Here's how the part is built. I have some questions about the finished solid (model axes, mm). Face numbers are marked on the shaded views. Round coordinates to 2 decimals unless told otherwise and drop trailing zeros. Write each loop counter-clockwise with the first axis right and the second up, starting at its lowest first coordinate (ties: lowest second). Pieces come first, ordered by that corner, then holes. Notation, with made-up numbers: (30, 81) -> (57, 81) arc R19 ccw to (57, 88) -> close; hole circle Ø7 at (21, 71.25). An arc over 180 degrees is marked (long way). Answer in a Markdown table with one row per item.
from build123d import *

# Parameters (mm, degrees)
CYLINDER_R       = 1.2
CYLINDER_DEPTH   = 10
ARRAY001_X_COUNT = 2
ARRAY001_X_PITCH = 29.6
ARRAY001_Y_COUNT = 2
ARRAY001_Y_PITCH = 17.8
BOX003_W         = 23.6
BOX003_H         = 11.8
BOX003_DEPTH     = 10
BOX002_W         = 35.6
BOX002_H         = 23.8
BOX002_DEPTH     = 2.5
BOX017_W         = 2.5
BOX017_H         = 23.8
BOX017_DEPTH     = 1.5
BOX005_W         = 35.6
BOX005_H         = 2.5
BOX005_DEPTH     = 1.5


with BuildPart() as bolt_hole_array_clone:
    # Cylinder → Cylinder (new body)
    with BuildSketch(Plane.XY):
        Circle(CYLINDER_R)
    extrude(amount=CYLINDER_DEPTH)

    # Array001 X: bolt hole array clone ×2


with BuildPart() as bolt_hole_array_clone_1:
    add(bolt_hole_array_clone.part)
    with Locations(*[(i * ARRAY001_X_PITCH, 0, 0) for i in range(1, ARRAY001_X_COUNT)]):
        add(bolt_hole_array_clone.part)

    # Array001 Y: bolt hole array clone ×2


with BuildPart() as bolt_hole_array_clone_2:
    add(bolt_hole_array_clone_1.part)
    with Locations(*[(0, i * ARRAY001_Y_PITCH, 0) for i in range(1, ARRAY001_Y_COUNT)]):
        add(bolt_hole_array_clone_1.part)


with BuildPart() as bolt_hole_array_clone_3:
    # Array001 placement: moved
    add(bolt_hole_array_clone_2.part.moved(Location((3, 3, 0))))


with BuildPart() as mesh_extraction_fusion:
    # Box003 → Box003 (new body)
    with BuildSketch(Plane(origin=(6, 6, 0), x_dir=(1, 0, 0), z_dir=(0, 0, 1))):
        with Locations((11.8, 5.9)):
            Rectangle(BOX003_W, BOX003_H)
    extrude(amount=BOX003_DEPTH)

    # Fusion003: union bolt hole array clone
    add(bolt_hole_array_clone_3.part)


with BuildPart() as mesh_border_cut:
    # Box002 → Box002 (new body)
    with BuildSketch(Plane.XY):
        with Locations((17.8, 11.9)):
            Rectangle(BOX002_W, BOX002_H)
    extrude(amount=BOX002_DEPTH)

    # Cut001: cut mesh extraction fusion
    add(mesh_extraction_fusion.part, mode=Mode.SUBTRACT)


with BuildPart() as obj1:
    # Box017 → Box017 (new body)
    with BuildSketch(Plane.XY):
        with Locations((1.25, 11.9)):
            Rectangle(BOX017_W, BOX017_H)
    extrude(amount=BOX017_DEPTH)


with BuildPart() as obj1_1:
    # Array011 placement: moved
    add(obj1.part.moved(Location((16.55, 0, 0))))


with BuildPart() as x_mesh_holder_fusion:
    # Box005 → Box005 (new body)
    with BuildSketch(Plane.XY):
        with Locations((17.8, 1.25)):
            Rectangle(BOX005_W, BOX005_H)
    extrude(amount=BOX005_DEPTH)


with BuildPart() as x_mesh_holder_fusion_1:
    # Array002 placement: moved
    add(x_mesh_holder_fusion.part.moved(Location((0, 10.65, 0))))

    # Fusion001: union mesh border cut, obj1
    add(mesh_border_cut.part)
    add(obj1_1.part)


solid = x_mesh_holder_fusion_1.part
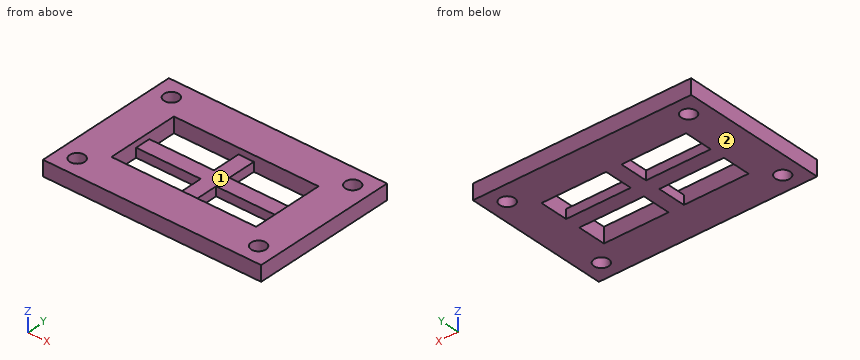
1) I want a section at C-C, the plane z = 0.45. Count the separate pieces of the cut face and the enclosed holes in it, and give its area (3 significant figures).
Response:
| item | result |
|---|---|
| separate pieces | 1 |
| enclosed holes | 8 |
| area | 633 mm^2 |
2) We'd pull the mould along Y, two halves only. Please class the marked faces 1 and 2: +Y half, -Y half, draft (parallel to the pull), parting line (faces both ways), or undercut.
Response:
| item | result |
|---|---|
| face 1 | undercut |
| face 2 | draft |
3) I need wall thicknesses on line 1 (Y direction, x = 12, z = 0.9); line 2 (X direction, y = 3, z = 1); line 3 (X direction, y = 6.5, z = 0.4). Which ranges of each line are inside material? Lowest first, please. Write a range as [from, to].
Response:
| item | result |
|---|---|
| line 1 | y = [0, 6], [10.65, 13.15], [17.8, 23.8] |
| line 2 | x = [0, 1.8], [4.2, 31.4], [33.8, 35.6] |
| line 3 | x = [0, 6], [16.55, 19.05], [29.6, 35.6] |
4) For pin 1 (3 mm diameter, centred on x = 32.6, y = 20.8, fed in from -Z); pin 2 (1.9 mm diameter, centred on x = 3, y = 3, fed in from +Z); pin 3 (3.5 mm diameter, centred on x = 18.5, y = 13, fed in from +Z), each with a flat end and sliding along its axis, tell me the tip position at first contact or that it passes through.
Response:
| item | result |
|---|---|
| pin 1 | stops at z = 0 |
| pin 2 | passes through |
| pin 3 | stops at z = 1.5 |
5) I want a section at A-A, the plane y = 3. List the corners of the cut face in (x, z) for me, and give its area (3 significant figures).
Response:
| item | result |
|---|---|
| outline | (0, 0) -> (1.8, 0) -> (1.8, 2.5) -> (0, 2.5) -> close; (4.2, 0) -> (31.4, 0) -> (31.4, 2.5) -> (4.2, 2.5) -> close; (33.8, 0) -> (35.6, 0) -> (35.6, 2.5) -> (33.8, 2.5) -> close |
| area | 77.0 mm^2 |
6) I want a section at B-B, the plane x = 26. List the corners of the cut face in (y, z) for me.
Response:
| item | result |
|---|---|
| outline | (0, 0) -> (6, 0) -> (6, 2.5) -> (0, 2.5) -> close; (10.65, 0) -> (13.15, 0) -> (13.15, 1.5) -> (10.65, 1.5) -> close; (17.8, 0) -> (23.8, 0) -> (23.8, 2.5) -> (17.8, 2.5) -> close |
7) I want a section at D-D, the plane x = 18. List the corners of the cut face in (y, z) for me.
Response:
| item | result |
|---|---|
| outline | (0, 0) -> (23.8, 0) -> (23.8, 2.5) -> (17.8, 2.5) -> (17.8, 1.5) -> (6, 1.5) -> (6, 2.5) -> (0, 2.5) -> close |
